```python
from build123d import *

# Parameters (mm, degrees)
SKETCH_2_W          = 10
SKETCH_2_H          = 22
CUT_EXTRUDE_1_DEPTH = 111.170322683
SKETCH_3_R          = 4
CUT_EXTRUDE_2_DEPTH = 102.002475217
CHAMFER_1_SIZE      = 2
CHAMFER_2_SIZE      = 1
CHAMFER_3_SIZE      = 0.5


with BuildPart() as part:
    # 草图1 → 旋转1 (revolve)
    with BuildSketch(Plane.XY, mode=Mode.PRIVATE) as revolve_1_sk:
        Polygon((0, 19), (0, 32.5), (10, 32.5), (10, 67.5), (22, 67.5), (22, 32.5), (55, 32.5), (55, 19), align=None)
    revolve(revolve_1_sk.sketch.rotate(Axis((0, 0, 0), (1, 0, 0)), 90), axis=Axis((0, 0, 0), (1, 0, 0)))

    # 草图2 → 切除-拉伸1 (cut, through all)
    with BuildSketch(Plane(origin=(55, 0, 0), x_dir=(0, 0, -1), z_dir=(1, 0, 0))):
        with Locations((0, 11)):
            Rectangle(SKETCH_2_W, SKETCH_2_H)
    extrude(amount=-CUT_EXTRUDE_1_DEPTH, mode=Mode.SUBTRACT)

    # 草图3 → 切除-拉伸2 (cut, through all)
    with BuildSketch(Plane(origin=(22, 0, 0), x_dir=(0, 0, -1), z_dir=(1, 0, 0))):
        with Locations((0, 57.5)):
            Circle(SKETCH_3_R)
        with Locations((40.658639918, 40.658639918)):
            Circle(SKETCH_3_R)
        with Locations((57.5, 0)):
            Circle(SKETCH_3_R)
        with Locations((40.658639918, -40.658639918)):
            Circle(SKETCH_3_R)
        with Locations((0, -57.5)):
            Circle(SKETCH_3_R)
        with Locations((-40.658639918, -40.658639918)):
            Circle(SKETCH_3_R)
        with Locations((-57.5, 0)):
            Circle(SKETCH_3_R)
        with Locations((-40.658639918, 40.658639918)):
            Circle(SKETCH_3_R)
    extrude(amount=-CUT_EXTRUDE_2_DEPTH, mode=Mode.SUBTRACT)

    # 倒角1
    chamfer_1_edges = [part.edges().sort_by_distance(p)[0] for p in [
        (22, 0, -67.5),
    ]]
    chamfer(chamfer_1_edges, length=CHAMFER_1_SIZE)

    # 倒角2
    chamfer_2_edges = [part.edges().sort_by_distance(p)[0] for p in [
        (0, -19, 0),
    ]]
    chamfer(chamfer_2_edges, length=CHAMFER_2_SIZE)

    # 倒角3
    chamfer_3_edges = [part.edges().sort_by_distance(p)[0] for p in [
        (55, -19, 0),
        (10, 57.5, 4),
        (22, 57.5, 4),
        (10, 40.658639918, -36.658639918),
        (22, 40.658639918, -36.658639918),
        (10, 0, -53.5),
        (22, 0, -53.5),
        (10, -40.658639918, -36.658639918),
        (22, -40.658639918, -36.658639918),
        (10, -57.5, 4),
        (22, -57.5, 4),
        (10, -40.658639918, 44.658639918),
        (22, -40.658639918, 44.658639918),
        (10, 0, 61.5),
        (22, 0, 61.5),
        (10, 40.658639918, 44.658639918),
        (22, 40.658639918, 44.658639918),
        (55, 0, -32.5),
        (10, 0, -67.5),
    ]]
    chamfer(chamfer_3_edges, length=CHAMFER_3_SIZE)


solid = part.part
```
Here's how the part is built. I have some questions about the finished solid (model axes, mm). A direction names the side the tool comes from. Coordinates: 2 decimals unless noted, no trailing zeros. Loops run counter-clockwise (first coordinate to the right, second up) from the corner with the lowest first, then second, coordinate; pieces in that order, holes last. Notation, with made-up numbers: (85.5, 85.25) - (130.5, 85.25) arc R16 cw to (130.5, 90.25) - close; hole circle Ø8 at (-33, -28). An arc over 180 degrees is marked (long way). Return JSON: item names as keys, results as strings. Group by question number.
Item 1: Will these pins go through, and if not, where does the flat tip stop? P1, Ø7, axis at y = 0, z = 57.5, coming from the -X side; P2, Ø1.8, axis at x = 18, y = 20, coming from the +Z side; P3, Ø2, axis at x = 21.5, z = 0.5, coming from the -Y side; P4, Ø3, axis at y = 16.5, z = -34, coming from the -X side.
Item 2: If we section it at A-A on x = 33: Write out the boundary of the cut face in (y, z), and give its area (3 significant figures).
Item 3: I need wall thicknesses on line 1 (Y direction, x = 14, z = 0); line 2 (X direction, y = 7, z = -33.5); line 3 (Z direction, x = 42, y = -11.5). Which ranges of each line are inside material? Lowest first, please. Write a range as from..to.
Item 4: If we section it at B-B on x = 14.5: State how many separate pieces and enclosed holes the cut face has, and give its area (3 significant figures).
Item 5: We'd pull the mould along Y, two halves only. Please class faces 3 (the face through (28, 20, -5)), 4 (the face through (38.48, -9.76, 31)), 5 (the face through (16.077, 1.201, -61.315)), 6 (the face through (55, -15, 14)): +Y half, -Y half, draft (parallel to the pull), parting line (faces both ways), or undercut.
Item 6: On a 3-axis mill with a long thin cutter (end or side, diameter ignored), from which of +Z, -Z, +X, -X, +Y, -Y can I reach the whole of each face in a straight line? I mean faces 1 (the face through (28, 22, 0)), 2 (the face through (5.07, -9.76, 31)). Say none if no direction works.
Calculated:
{
 "1": {"P1": "passes through", "P2": "stops at z = 64.74", "P3": "stops at y = -67", "P4": "stops at x = 10"},
 "2": {"outline": "circle Ø65 at (0, 0); hole (18.33, -5) - (22, -5) - (22, 5) - (18.33, 5) arc R19 ccw (long way) to start", "area": "2,150 mm^2"},
 "3": {"line 1": "y = -67.5..-61.5, -53.5..-19, 22..53.5, 61.5..67.5", "line 2": "x = 10..22", "line 3": "z = -30.4..-15.12, 15.12..30.4"},
 "4": {"separate pieces": "1", "enclosed holes": "9", "area": "12,700 mm^2"},
 "5": {"face 3": "undercut", "face 4": "parting line", "face 5": "undercut", "face 6": "draft"},
 "6": {"face 1": "+X, -X", "face 2": "-X"}
}
